Geometry: final body of the model. Coordinates: model frame, mm. Give positions to 0.01 mm unless a question says otherwise; leave off trailing zeros. Loops run counter-clockwise (first coordinate to the right, second up) from the corner with the lowest first, then second, coordinate; pieces in that order, holes last. Notation, with made-up numbers: (-39, -38) - (-1, -38) arc R17 ccw to (-1, -14) - close; hole circle Ø8 at (51.5, 17.5). An arc over 180 degrees is marked (long way). Answer in a Markdown table with one row per item.
from build123d import *

# Parameters (mm, degrees)
EXTRUDE_1_DEPTH         = 3
EXTRUDE_START           = -42
EXTRUDE_2_OUTLINE_W     = 3
EXTRUDE_2_OUTLINE_H     = 100
EXTRUDE_2_DEPTH         = 41
EXTRUDE_START_2         = -1
EXTRUDE_2_2_OUTLINE_R   = 2
EXTRUDE_2_2_OUTLINE_W   = 10
EXTRUDE_2_2_OUTLINE_H   = 120
EXTRUDE_2_2_OUTLINE_R_2 = 52
EXTRUDE_2_2_DEPTH       = 4
EXTRUDE_START_3         = -47
EXTRUDE_2_3_OUTLINE_W   = 3
EXTRUDE_2_3_OUTLINE_H   = 100
EXTRUDE_2_3_DEPTH       = 5
EXTRUDE_2_4_DEPTH       = 180
EXTRUDE_START_4         = -5
EXTRUDE_2_5_DEPTH       = 5
EXTRUDE_START_5         = -3
SKETCH_3_R              = 52
SKETCH_3_W              = 10
SKETCH_3_H              = 120
EXTRUDE_3_DEPTH         = 3
SKETCH_4_R              = 2
EXTRUDE_4_DEPTH         = 3
EXTRUDE_START_6         = -56
SKETCH_5_R              = 2
EXTRUDE_5_DEPTH         = 56
SKETCH_6_W              = 375.582573206
SKETCH_6_H              = 223.737414549
CUT_EXTRUDE_1_DEPTH     = 70
CUT_EXTRUDE_2_DEPTH     = 126
SKETCH_8_W              = 410.596490254
SKETCH_8_H              = 121.986596881
CUT_EXTRUDE_3_DEPTH     = 10
SKETCH_9_W              = 309.492357762
SKETCH_9_H              = 10
EXTRUDE_6_DEPTH         = 3
SKETCH_10_W             = 76.162490496
SKETCH_10_H             = 157.997962214
CUT_EXTRUDE_4_DEPTH     = 10


with BuildPart() as part:
    # 草图1 → 凸台-拉伸1 (new body)
    with BuildSketch(Plane(origin=(-1, 0, 0), x_dir=(0, 0, -1), z_dir=(1, 0, 0))):
        Polygon((33.371794872, 92.353263785), (31.902170139, 91.718942203), (33.371794872, 91.084620622), align=None)
    extrude(amount=-EXTRUDE_1_DEPTH)

    # 凸台-拉伸2: read off the stored shape, not the designer's step
    # 凸台-拉伸2 outline → 凸台-拉伸2 (add)
    with BuildSketch(Plane.XY.offset(EXTRUDE_START)):
        with Locations((-2.5, 90)):
            Rectangle(EXTRUDE_2_OUTLINE_W, EXTRUDE_2_OUTLINE_H)
    extrude(amount=EXTRUDE_2_DEPTH)

    # Extrude 2 2 outline → Extrude 2 2 (add)
    with BuildSketch(Plane.XY.offset(EXTRUDE_START_2)):
        with BuildLine():
            Line((-4, 140), (-4, 40))
            Line((-4, 40), (0, 40))
            ThreePointArc((0, 40), (11.715728753, 11.715728753), (40, 0))
            Line((40, 0), (220, 0))
            ThreePointArc((220, 0), (310, 90), (220, 180))
            Line((220, 180), (40, 180))
            ThreePointArc((40, 180), (11.715728753, 168.284271247), (0, 140))
            Line((0, 140), (-4, 140))
        make_face()
        with Locations((248.3, 165.059930776)):
            Circle(EXTRUDE_2_2_OUTLINE_R, mode=Mode.SUBTRACT)
        with Locations((28, 14)):
            Circle(EXTRUDE_2_2_OUTLINE_R, mode=Mode.SUBTRACT)
        with Locations((139.15, 14)):
            Circle(EXTRUDE_2_2_OUTLINE_R, mode=Mode.SUBTRACT)
        with Locations((27.7366, 79.2634)):
            Circle(EXTRUDE_2_2_OUTLINE_R, mode=Mode.SUBTRACT)
        with Locations((248.3, 14.940069224)):
            Circle(EXTRUDE_2_2_OUTLINE_R, mode=Mode.SUBTRACT)
        with Locations((27.7366, 104.2634)):
            Circle(EXTRUDE_2_2_OUTLINE_R, mode=Mode.SUBTRACT)
        with Locations((107.15, 90)):
            Rectangle(EXTRUDE_2_2_OUTLINE_W, EXTRUDE_2_2_OUTLINE_H, mode=Mode.SUBTRACT)
        with Locations((137.15, 90)):
            Rectangle(EXTRUDE_2_2_OUTLINE_W, EXTRUDE_2_2_OUTLINE_H, mode=Mode.SUBTRACT)
        with Locations((28, 166)):
            Circle(EXTRUDE_2_2_OUTLINE_R, mode=Mode.SUBTRACT)
        with Locations((139.15, 166)):
            Circle(EXTRUDE_2_2_OUTLINE_R, mode=Mode.SUBTRACT)
        with Locations((220, 90)):
            Circle(EXTRUDE_2_2_OUTLINE_R_2, mode=Mode.SUBTRACT)
    extrude(amount=EXTRUDE_2_2_DEPTH)

    # Extrude 2 3 outline → Extrude 2 3 (add)
    with BuildSketch(Plane.XY.offset(EXTRUDE_START_3)):
        with Locations((-2.5, 90)):
            Rectangle(EXTRUDE_2_3_OUTLINE_W, EXTRUDE_2_3_OUTLINE_H)
    extrude(amount=EXTRUDE_2_3_DEPTH)

    # Extrude 2 4 outline → Extrude 2 4 (cut)
    with BuildSketch(Plane(origin=(0, 0, 0), x_dir=(1, 0, 0), z_dir=(0, 1, 0))):
        with BuildLine():
            Line((311, 0), (311, 1))
            Line((311, 1), (-1, 1))
            ThreePointArc((-1, 1), (-0.707106781, 0.292893219), (0, 0))
            Line((0, 0), (311, 0))
        make_face()
        with BuildLine():
            Line((102.15, -4), (102.15, -3))
            Line((102.15, -3), (0, -3))
            ThreePointArc((0, -3), (-2.828427125, -1.828427125), (-4, 1))
            Line((-4, 1), (-4, 2))
            Line((-4, 2), (-5, 2))
            Line((-5, 2), (-5, -4))
            Line((-5, -4), (102.15, -4))
        make_face()
    extrude(amount=EXTRUDE_2_4_DEPTH, mode=Mode.SUBTRACT)

    # Extrude 2 5 outline → Extrude 2 5 (cut)
    with BuildSketch(Plane.YZ.offset(EXTRUDE_START_4)):
        with BuildLine():
            ThreePointArc((45, -47), (41.464466094, -45.535533906), (40, -42))
            Line((40, -42), (40, -41))
            Line((40, -41), (39, -41))
            Line((39, -41), (39, -46.999999996))
            Line((39, -46.999999996), (45, -47))
        make_face()
        with BuildLine():
            ThreePointArc((140, -42), (138.535533906, -45.535533906), (135, -47))
            Line((135, -47), (141, -46.999999996))
            Line((141, -46.999999996), (141, -41))
            Line((141, -41), (140, -41))
            Line((140, -41), (140, -42))
        make_face()
    extrude(amount=EXTRUDE_2_5_DEPTH, mode=Mode.SUBTRACT)

    # 草图3 → 凸台-拉伸3 (add)
    with BuildSketch(Plane.XY.offset(3).offset(EXTRUDE_START_5)):
        with Locations((220, 90)):
            Circle(SKETCH_3_R)
        with Locations((107.15, 90)):
            Rectangle(SKETCH_3_W, SKETCH_3_H)
        with Locations((137.15, 90)):
            Rectangle(SKETCH_3_W, SKETCH_3_H)
    extrude(amount=EXTRUDE_3_DEPTH)

    # 草图4 → 凸台-拉伸4 (add)
    with BuildSketch(Plane.XY.offset(3).offset(EXTRUDE_START_5)):
        with Locations((27.7366, 79.2634)):
            Circle(SKETCH_4_R)
        with Locations((27.7366, 104.2634)):
            Circle(SKETCH_4_R)
    extrude(amount=EXTRUDE_4_DEPTH)

    # 草图5 → 凸台-拉伸5 (add)
    with BuildSketch(Plane.XY.offset(3).offset(EXTRUDE_START_6)):
        with Locations((248.3, 14.940069224)):
            Circle(SKETCH_5_R)
        with Locations((139.15, 14)):
            Circle(SKETCH_5_R)
        with Locations((248.3, 165.059930776)):
            Circle(SKETCH_5_R)
        with Locations((139.15, 166)):
            Circle(SKETCH_5_R)
        with Locations((28, 14)):
            Circle(SKETCH_5_R)
        with Locations((28, 166)):
            Circle(SKETCH_5_R)
    extrude(amount=EXTRUDE_5_DEPTH)

    # 草图6 → 切除-拉伸1 (cut)
    with BuildSketch(Plane(origin=(0, 0, 0), x_dir=(-1, 0, 0), z_dir=(0, 0, -1))):
        with Locations((-149.296459545, 93.267829814)):
            Rectangle(SKETCH_6_W, SKETCH_6_H)
    extrude(amount=CUT_EXTRUDE_1_DEPTH, mode=Mode.SUBTRACT)

    # 草图7 → 切除-拉伸2 (cut)
    with BuildSketch(Plane.XZ.offset(-40)):
        with BuildLine():
            Line((-3.872983346, 0), (0, 0))
            Line((0, 0), (0, 3))
            ThreePointArc((0, 3), (-2.449489743, 2.16227766), (-3.872983346, 0))
        make_face()
    extrude(amount=-CUT_EXTRUDE_2_DEPTH, mode=Mode.SUBTRACT)

    # 草图8 → 切除-拉伸3 (cut)
    with BuildSketch(Plane(origin=(0, 0, 0), x_dir=(-1, 0, 0), z_dir=(0, 0, -1))):
        with Locations((-160.461750975, 150.993298441)):
            Rectangle(SKETCH_8_W, SKETCH_8_H)
    extrude(amount=-CUT_EXTRUDE_3_DEPTH, mode=Mode.SUBTRACT)

    # 草图9 → 凸台-拉伸6 (add)
    with BuildSketch(Plane(origin=(0, 0, 0), x_dir=(-1, 0, 0), z_dir=(0, 0, -1))):
        with Locations((-154.746178881, 95)):
            Rectangle(SKETCH_9_W, SKETCH_9_H)
    extrude(amount=-EXTRUDE_6_DEPTH)

    # 镜向1: part across plane


with BuildPart() as part_1:
    add(part.part)
    add(part.part.mirror(Plane(origin=(309.492357762, 100, 312.653870495), x_dir=(0, 0, 1), z_dir=(0, 1, 0))))

    # 草图10 → 切除-拉伸4 (cut)
    with BuildSketch(Plane(origin=(0, 0, 0), x_dir=(-1, 0, 0), z_dir=(0, 0, -1))):
        with Locations((-338.081245248, 107.574371838)):
            Rectangle(SKETCH_10_W, SKETCH_10_H)
    extrude(amount=-CUT_EXTRUDE_4_DEPTH, mode=Mode.SUBTRACT)


solid = part_1.part
Q1. Cut plane A-A (z = 1.7). Output: boundary loops of the cut face in (x, y), and give its area (3 significant figures).
Check values:
| item | result |
|---|---|
| outline | (0, 40) arc R40 ccw to (40, 0) - (220, 0) arc R90 ccw to (300, 48.77) - (300, 151.23) arc R90 ccw to (220, 200) - (40, 200) arc R40 ccw to (0, 160) - close |
| area | 57,100 mm² |
Q2. Material intervals for line 1 along Y through (x, z) = (31, 1.9); line 2 along X through (y, z) = (39, 2.85); line 3 along X through (y, z) = (153, 2.3), sorted ascending.
Check values:
| item | result |
|---|---|
| line 1 | 1.03 to 198.97 |
| line 2 | 0.01 to 294.16 |
| line 3 | 0 to 299.06 |
Q3. Cut plane B-B (y = 175.5). Output: boundary loops of the cut face in (x, z), and give its area (3 significant figures).
Check values:
| item | result |
|---|---|
| outline | (3.13, 0) - (281.72, 0) - (281.72, 3) - (3.13, 3) - close |
| area | 836 mm² |
Q4. Cut plane C-C (x = 268). Output: boundary loops of the cut face in (y, z), and give its area (3 significant figures).
Check values:
| item | result |
|---|---|
| outline | (13.87, 0) - (186.13, 0) - (186.13, 3) - (13.87, 3) - close |
| area | 517 mm² |
Q5. First-contact query: pin 1 (1.5 mm diameter, centred on y = 36, z = 1, fed in from +X). Flat tip, straight axial feed; report the tip coordinate or a pass-through.
Check values:
| item | result |
|---|---|
| pin 1 | x = 292.56 |
